The listing builds one solid part. Answer for the finished solid, in the listing's coordinates (mm). Face numbers are marked on the shaded views. A direction names the side the tool comes from. Coordinates: 2 decimals unless noted, no trailing zeros. Loops run counter-clockwise (first coordinate to the right, second up) from the corner with the lowest first, then second, coordinate; pieces in that order, holes last. Notation, with made-up numbers: M 71,-23.5 L 101,-23.5 A21 cw 101,-9.5 Z; hole C 66.25,-15 d9. An arc over 180 degrees is marked long. Return JSON: item names as keys, results as strings. Group by question number.
1. Section C-C (z = 26) is taken. Write down the section's boundary in (x, y), then the cut area to 3 significant figures.
2. Given P1, Ø12, axis at x = -17.5, y = -42.5, coming from the +Z side; P2, Ø11, axis at x = 21, z = 18, coming from the +Y side; P3, Ø2.5, axis at x = -40, z = 10, coming from the +Y side, each flat-ended and moving along its own axis, determine where each tip first touches the part or whether it passes through.
3. Straight lines are drawn through the part: L1, parallel to X at y = -53.8, z = 10; L2, parallel to Y at x = 0, z = 9; L3, parallel to Y at x = -8.25, z = 13.75. For each, find the intervals that lie inside material, in ascending order. Write a range as from..to.
4. Section D-D (y = -17) is taken. Write down the section's boundary in (x, z), then the cut area to 3 significant figures.
5. Which of the six approach directions +Z, -Z, +X, -X, +Y, -Y give full straight-line access (tool end or side, diameter ignored) to the marked faces 1, 2, 3, 4 and 5?
6. Section A-A (y = 25) is taken. Write down the section's boundary in (x, z).
7. Section B-B (x = 8.25) is taken. Write down the section's boundary in (y, z), then the cut area to 3 significant figures.
8. The mould has two halves that part along Y. Classify the marked faces 6, 7 and 8: pulls with the +Y half, pulls with the -Y half, needs draft (parallel to the pull), parting line crosses it, or undercut.
```python
from build123d import *

# Parameters (mm, degrees)
SKETCH_1_W                 = 96
SKETCH_1_H                 = 110
EXTRUDE_1_DEPTH            = 20
CUT_EXTRUDE_1_DEPTH        = 20
SHELL_1_T                  = -4
SHELL_1_THICKNESS_2_FACE_W = 16
SHELL_1_THICKNESS_2_FACE_H = 52
SHELL_1_THICKNESS_2_DEPTH  = 36
CUT_EXTRUDE_2_REACH        = 123.672
SKETCH_3_R                 = 2
CUT_EXTRUDE_3_REACH        = 77.69
SKETCH_5_R                 = 2.5
SKETCH_6_W                 = 96
SKETCH_6_H                 = 20
EXTRUDE_2_DEPTH            = 4
EXTRUDE_3_DEPTH            = 4
FILLET_1_R                 = 3
CUT_EXTRUDE_4_DEPTH        = 2.4
SKETCH_10_W                = 8
SKETCH_10_H                = 8
CUT_EXTRUDE_5_DEPTH        = 104.484298326
FILLET_2_R                 = 2
CHAMFER_1_SIZE             = 3


with BuildPart() as part:
    # 草图1 → 凸台-拉伸1 (new body)
    with BuildSketch(Plane.XY):
        Rectangle(SKETCH_1_W, SKETCH_1_H)
    extrude(amount=EXTRUDE_1_DEPTH)

    # 草图2 → 切除-拉伸1 (cut)
    with BuildSketch(Plane.XY.offset(20)):
        Polygon((-48, -30), (-30, 1.176914536), (-30, 55), (-48, 55), align=None)
        Polygon((48, 55), (48, -30), (30, 1.176914536), (30, 55), align=None)
    extrude(amount=-CUT_EXTRUDE_1_DEPTH, mode=Mode.SUBTRACT)

    # 抽壳1
    shell_1_openings = [part.faces().sort_by_distance(p)[0] for p in [
        (0, -6.109962386, 20),
    ]]
    offset(amount=SHELL_1_T, openings=shell_1_openings, kind=Kind.INTERSECTION)

    # 抽壳1 thickness 2 face (on inner face of the shell) → 抽壳1 thickness 2 (add)
    with BuildSketch(Plane(origin=(0, 51, 12), x_dir=(0, 0, 1), z_dir=(0, 1, 0))):
        Rectangle(SHELL_1_THICKNESS_2_FACE_W, SHELL_1_THICKNESS_2_FACE_H)
    extrude(amount=-SHELL_1_THICKNESS_2_DEPTH)

    # 草图3 → 切除-拉伸2 (cut, up to next)
    with BuildSketch(Plane.XZ.offset(55), mode=Mode.PRIVATE) as cut_extrude_2_sk1:
        with Locations(Location((-40, 10, 0), (0, 0, 270))):
            Circle(SKETCH_3_R)
    cut_extrude_2_tool1 = extrude(cut_extrude_2_sk1.sketch, amount=-CUT_EXTRUDE_2_REACH, mode=Mode.PRIVATE) & part.part
    # 草图3 → 切除-拉伸2 (cut, up to next)
    with BuildSketch(Plane.XZ.offset(55), mode=Mode.PRIVATE) as cut_extrude_2_sk2:
        with Locations(Location((40, 10, 0), (0, 0, 270))):
            Circle(SKETCH_3_R)
    cut_extrude_2_tool2 = extrude(cut_extrude_2_sk2.sketch, amount=-CUT_EXTRUDE_2_REACH, mode=Mode.PRIVATE) & part.part
    add(cut_extrude_2_tool1.solids().sort_by_distance((-40, -55, 10))[0], mode=Mode.SUBTRACT)
    add(cut_extrude_2_tool2.solids().sort_by_distance((40, -55, 10))[0], mode=Mode.SUBTRACT)

    # 草图5 → 切除-拉伸3 (cut, up to next)
    with BuildSketch(Plane.XY.offset(20), mode=Mode.PRIVATE) as cut_extrude_3_sk1:
        with Locations((0, 25)):
            Circle(SKETCH_5_R)
    cut_extrude_3_tool1 = extrude(cut_extrude_3_sk1.sketch, amount=-CUT_EXTRUDE_3_REACH, mode=Mode.PRIVATE) & part.part
    # 草图5 → 切除-拉伸3 (cut, up to next)
    with BuildSketch(Plane.XY.offset(20), mode=Mode.PRIVATE) as cut_extrude_3_sk2:
        with Locations((-8.25, 35.046765649)):
            Circle(SKETCH_5_R)
    cut_extrude_3_tool2 = extrude(cut_extrude_3_sk2.sketch, amount=-CUT_EXTRUDE_3_REACH, mode=Mode.PRIVATE) & part.part
    # 草图5 → 切除-拉伸3 (cut, up to next)
    with BuildSketch(Plane.XY.offset(20), mode=Mode.PRIVATE) as cut_extrude_3_sk3:
        with Locations(Location((8.25, 35.046765649, 0), (0, 0, 180))):
            Circle(SKETCH_5_R)
    cut_extrude_3_tool3 = extrude(cut_extrude_3_sk3.sketch, amount=-CUT_EXTRUDE_3_REACH, mode=Mode.PRIVATE) & part.part
    add(cut_extrude_3_tool1.solids().sort_by_distance((0, 25, 20))[0], mode=Mode.SUBTRACT)
    add(cut_extrude_3_tool2.solids().sort_by_distance((-8.25, 35.046766, 20))[0], mode=Mode.SUBTRACT)
    add(cut_extrude_3_tool3.solids().sort_by_distance((8.25, 35.046766, 20))[0], mode=Mode.SUBTRACT)

    # 草图6 → 凸台-拉伸2 (add)
    with BuildSketch(Plane.XZ.offset(55)):
        with Locations((0, 30)):
            Rectangle(SKETCH_6_W, SKETCH_6_H)
    extrude(amount=-EXTRUDE_2_DEPTH)

    # 草图7 → 凸台-拉伸3 (add)
    with BuildSketch(Plane.ZY.offset(48)):
        Polygon((20, -36), (35, -44), (35, -51), (20, -51), align=None)
    extrude_3 = extrude(amount=-EXTRUDE_3_DEPTH)

    # 镜向1: 凸台-拉伸3 across plane
    add(extrude_3.mirror(Plane(origin=(0, 0, 0), x_dir=(0, 0, 1), z_dir=(1, 0, 0))))

    # 圆角1
    fillet_1_edges = [part.edges().sort_by_distance(p)[0] for p in [
        (-48, -53, 40),
        (48, -53, 40),
    ]]
    fillet(fillet_1_edges, radius=FILLET_1_R)

    # 草图8 → 切除-拉伸4 (cut)
    with BuildSketch(Plane(origin=(0, -51, 0), x_dir=(1, 0, 0), z_dir=(0, 1, 0))):
        Polygon((40, -13.348631561), (42.9, -11.674315781), (42.9, -8.325684219), (40, -6.651368439), (37.1, -8.325684219), (37.1, -11.674315781), align=None)
        Polygon((-37.1, -11.674315781), (-40, -13.348631561), (-42.9, -11.674315781), (-42.9, -8.325684219), (-40, -6.651368439), (-37.1, -8.325684219), align=None)
    extrude(amount=-CUT_EXTRUDE_4_DEPTH, mode=Mode.SUBTRACT)

    # 草图10 → 切除-拉伸5 (cut, through all)
    with BuildSketch(Plane.ZY.offset(30)):
        with Locations((16, 51)):
            Rectangle(SKETCH_10_W, SKETCH_10_H)
    extrude(amount=-CUT_EXTRUDE_5_DEPTH, mode=Mode.SUBTRACT)

    # 圆角2
    fillet_2_edges = [part.edges().sort_by_distance(p)[0] for p in [
        (0, 47, 12),
    ]]
    fillet(fillet_2_edges, radius=FILLET_2_R)

    # 倒角1
    chamfer_1_edges = [part.edges().sort_by_distance(p)[0] for p in [
        (0, 55, 12),
    ]]
    chamfer(chamfer_1_edges, length=CHAMFER_1_SIZE)


solid = part.part
```
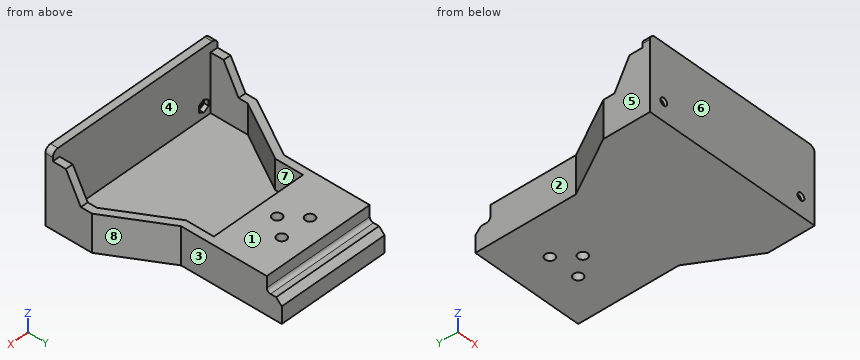
Worked out:
{
 "1": {"outline": "M -48,-55 L 48,-55 L 48,-39.2 L 44,-39.2 L 44,-51 L -44,-51 L -44,-39.2 L -48,-39.2 Z", "area": "478 mm^2"},
 "2": {"P1": "z = 4", "P2": "y = 47.68", "P3": "y = -13.98"},
 "3": {"L1": "-48..-42, -38..38, 42..48", "L2": "-55..-51, 15..22.5, 27.5..55", "L3": "-55..-51, 15..32.55, 37.55..47.02"},
 "4": {"outline": "M -40.49,0 L 40.49,0 L 40.49,20 L 35.88,20 L 35.88,4 L -35.88,4 L -35.88,20 L -40.49,20 Z", "area": "472 mm^2"},
 "5": {"face 1": "+Z, +X, -X, +Y", "face 2": "+Z, -Z, -X, +Y", "face 3": "+Z, -Z, +X, +Y", "face 4": "+Z", "face 5": "+Z, -Z, -X, +Y, -Y"},
 "6": {"outline": "M -30,0 L -2.5,0 L -2.5,20 L -30,20 Z; M 2.5,0 L 30,0 L 30,20 L 2.5,20 Z"},
 "7": {"outline": "M -55,0 L 32.55,0 L 32.55,20 L 15,20 L 15,4 L -51,4 L -51,40 L -55,40 Z; M 37.55,0 L 55,0 L 55,9 L 52,12 L 49,12 A2 cw 47,14 L 47,20 L 37.55,20 Z", "area": "1,060 mm^2"},
 "8": {"face 6": "pulls with the -Y half", "face 7": "undercut", "face 8": "pulls with the +Y half"}
}
